```python
from build123d import *

# Parameters (mm, degrees)
BOSS_EXTRUDE1_DEPTH = 3
SKETCH2_W           = 3
SKETCH2_H           = 10
SKETCH2_W_2         = 30
SKETCH2_H_2         = 3
BOSS_EXTRUDE2_DEPTH = 3
CUT_EXTRUDE1_DEPTH  = 10
SKETCH4_W           = 3
SKETCH4_H           = 10
SKETCH4_H_2         = 16.31
CUT_EXTRUDE2_DEPTH  = 10
SKETCH5_W           = 3
SKETCH5_H           = 13.703534411
SKETCH5_H_2         = 13.791377581
CUT_EXTRUDE3_DEPTH  = 10
SKETCH6_R           = 6.665876203
SKETCH6_R_2         = 6.014739453
SKETCH6_R_3         = 4.167493344
SKETCH6_R_4         = 7.942691131
SKETCH6_R_5         = 4.658905865
CUT_EXTRUDE4_DEPTH  = 10


with BuildPart() as part:
    # Sketch1 → Boss-Extrude1 (new body)
    with BuildSketch(Plane(origin=(0, 0, 0), x_dir=(0, 0, -1), z_dir=(1, 0, 0))):
        Polygon((-383, 12.016330065), (-84.3, 0), (0, 0), (0, 32.31), (-383, 32.31), align=None)
    extrude(amount=BOSS_EXTRUDE1_DEPTH)

    # Sketch2 → Boss-Extrude2 (add)
    with BuildSketch(Plane(origin=(3, 0, 0), x_dir=(0, 0, -1), z_dir=(1, 0, 0))):
        with Locations((-384.5, 22.016330065)):
            Rectangle(SKETCH2_W, SKETCH2_H)
        with Locations((-335, 33.81)):
            Rectangle(SKETCH2_W_2, SKETCH2_H_2)
        with Locations((-40, 33.81)):
            Rectangle(SKETCH2_W_2, SKETCH2_H_2)
        with Locations((-185, 33.81)):
            Rectangle(SKETCH2_W_2, SKETCH2_H_2)
    extrude(amount=-BOSS_EXTRUDE2_DEPTH)

    # Sketch3 → Cut-Extrude1 (cut)
    with BuildSketch(Plane(origin=(3, 0, 0), x_dir=(0, 0, -1), z_dir=(1, 0, 0))):
        with BuildLine():
            Line((-360.908901745, 27.636018628), (-300.908901745, 26.724931053))
            ThreePointArc((-300.908901745, 26.724931053), (-295.000691614, 20.634524412), (-301.091098255, 14.726314282))
            Line((-301.091098255, 14.726314282), (-361.091098255, 15.637401857))
            ThreePointArc((-361.091098255, 15.637401857), (-366.999308386, 21.727808498), (-360.908901745, 27.636018628))
        make_face()
        with BuildLine():
            Line((-268.447308122, 27.232123759), (-208.447308122, 26.321036184))
            ThreePointArc((-208.447308122, 26.321036184), (-201.554396303, 19.215561769), (-208.659870718, 12.32264995))
            Line((-208.659870718, 12.32264995), (-268.659870718, 13.233737525))
            ThreePointArc((-268.659870718, 13.233737525), (-275.552782537, 20.33921194), (-268.447308122, 27.232123759))
        make_face()
        with BuildLine():
            Line((-172.817042181, 26.780113256), (-112.817042181, 25.869025681))
            ThreePointArc((-112.817042181, 25.869025681), (-104.939428674, 17.748483493), (-113.059970863, 9.870869986))
            Line((-113.059970863, 9.870869986), (-173.059970863, 10.781957561))
            ThreePointArc((-173.059970863, 10.781957561), (-180.93758437, 18.902499749), (-172.817042181, 26.780113256))
        make_face()
    extrude(amount=-CUT_EXTRUDE1_DEPTH, mode=Mode.SUBTRACT)

    # Sketch4 → Cut-Extrude2 (cut)
    with BuildSketch(Plane(origin=(3, 0, 0), x_dir=(0, 0, -1), z_dir=(1, 0, 0))):
        with Locations((-81.5, 27.31)):
            Rectangle(SKETCH4_W, SKETCH4_H)
        with Locations((-74.5, 8.155)):
            Rectangle(SKETCH4_W, SKETCH4_H_2)
    extrude(amount=-CUT_EXTRUDE2_DEPTH, mode=Mode.SUBTRACT)

    # Sketch5 → Cut-Extrude3 (cut)
    with BuildSketch(Plane(origin=(3, 0, 0), x_dir=(0, 0, -1), z_dir=(1, 0, 0))):
        with Locations((-1.5, 31.851767205)):
            Rectangle(SKETCH5_W, SKETCH5_H)
        with Locations((-1.5, 0.104311209)):
            Rectangle(SKETCH5_W, SKETCH5_H_2)
    extrude(amount=-CUT_EXTRUDE3_DEPTH, mode=Mode.SUBTRACT)

    # Sketch6 → Cut-Extrude4 (cut)
    with BuildSketch(Plane(origin=(3, 0, 0), x_dir=(0, 0, -1), z_dir=(1, 0, 0))):
        with Locations((-375.865428414, 21.928511603)):
            Circle(SKETCH6_R)
        with Locations((-285.544135062, 25.435251305)):
            Circle(SKETCH6_R_2)
        with Locations((-280.443646207, 13.449102496)):
            Circle(SKETCH6_R_3)
        with Locations((-291.558874515, 13.83163916)):
            Circle(SKETCH6_R_3)
        with Locations((-191.057579024, 24.542665756)):
            Circle(SKETCH6_R_4)
        with Locations((-186.614565866, 10.842366657)):
            Circle(SKETCH6_R_5)
        with Locations((-198.037933391, 11.447109955)):
            Circle(SKETCH6_R_5)
    extrude(amount=-CUT_EXTRUDE4_DEPTH, mode=Mode.SUBTRACT)


solid = part.part
```
Can you work these out from the model? Positions are in its coordinate system, mm. A direction names the side the tool comes from. Coordinates: 2 decimals unless noted, no trailing zeros. Order: outer loops, then holes, each group sorted by start corner. A loop starts at its lowest first (then second) coordinate and runs counter-clockwise, first axis right, second up.
1. I'm going to push flat-ended pins straight in: pin 1 (10.5 mm diameter, centred on y = 11.45, z = 198.04, fed in from +X); pin 2 (0.9 mm diameter, centred on x = 1.5, z = 71.5, fed in from +Y); pin 3 (1.5 mm diameter, centred on x = 1.5, z = 385, fed in from +Y); pin 4 (8 mm diameter, centred on y = 20, z = 247.5, fed in from +X). Where does each tip first touch, or does it pass through?
2. For faces 4 (the face through (1.5, 20.8, 295)), 5 (the face through (3, 10, 153)), which set-ups out of +Z, -Z, +X, -X, +Y, -Y let a thin tool reach every point of the face, with its end or its side?
3. If we section it at B-B (z = 330.5): Please give me the cut outline in (x, y).
4. If we section it at C-C (x = 0.5): Give the number of separate pieces and of enclosed holes in the cut face, then the cut area to 3 significant figures.
5. If we section it at A-A (z = 153.5): Please give me the cut outline in (x, y).
6. I need wall thicknesses on line 1 (Z direction, x = 0.25, y = 30.5); line 2 (Y direction, x = 0.2, z = 106.5); line 3 (Y direction, x = 2, z = 18.5). Which ranges of each line are inside material? Lowest first, please.
7. Thinking about a two-plate mould opening in Z: for faces 1 (the face through (1.52, 18.73, 180.94)), 2 (the face through (1.479, 6.092, 235.741)), 3 (the face through (0, 10, 153)), which applies, +Z half, -Z half, draft (parallel to the pull), parting line (faces both ways), or undercut?
Entries:
1. pin 1: stops at x = 3
1. pin 2: stops at y = 32.31
1. pin 3: stops at y = 27.02
1. pin 4: passes through
2. face 4: +X, -X
2. face 5: +Z, -Z, +X, +Y, -Y
3. outline: (0, 9.9) - (3, 9.9) - (3, 15.17) - (0, 15.17) - close; (0, 27.17) - (3, 27.17) - (3, 35.31) - (0, 35.31) - close
4. separate pieces: 1
4. enclosed holes: 10
4. area: 7,070 mm2
5. outline: (0, 2.78) - (3, 2.78) - (3, 10.48) - (0, 10.48) - close; (0, 26.49) - (3, 26.49) - (3, 32.31) - (0, 32.31) - close
6. line 1: z = 3 to 80, 83 to 185.8, 196.31 to 282.3, 288.79 to 383
6. line 2: y = 0.89 to 13.12, 22.62 to 32.31
6. line 3: y = 0 to 32.31
7. face 1: undercut
7. face 2: +Z half
7. face 3: draft
